Geometry: final body of the model. Coordinates: model frame, mm. Face numbers are marked on the shaded views. A direction names the side the tool comes from. Round coordinates to 2 decimals unless told otherwise and drop trailing zeros. Loops run counter-clockwise (first coordinate to the right, second up) from the corner with the lowest first, then second, coordinate; pieces in that order, holes last. Notation, with made-up numbers: M -10.5,-35.5 L -1.5,-35.5 A21 cw -1.5,-7.5 Z; hole C 30.5,-40 d4. An arc over 180 degrees is marked long. Answer as a JSON object with one key per item and string values.
```python
from build123d import *

# Parameters (mm, degrees)
F2_R = 1.6002
F3_R = 5.08


with BuildPart() as f1:
    # F0 (on Front) → F1 (revolve)
    with BuildSketch(Plane.XZ):
        Polygon((6.985, 12.7), (6.985, 0), (20.6375, 0), (20.6375, 17.4625), (19.05, 17.4625), (19.05, 19.05), (17.4625, 19.05), (17.4625, 12.7), align=None)
    revolve(axis=Axis((0, 0, 17.878274), (0, 0, 1)))

    # F2
    f2_edges = [f1.edges().sort_by_distance(p)[0] for p in [
        (-17.4625, 0, 12.7),
        (-20.6375, 0, 0),
    ]]
    fillet(f2_edges, radius=F2_R)

    # F3
    f3_edges = [f1.edges().sort_by_distance(p)[0] for p in [
        (-6.985, 0, 12.7),
    ]]
    fillet(f3_edges, radius=F3_R)


solid = f1.part
```
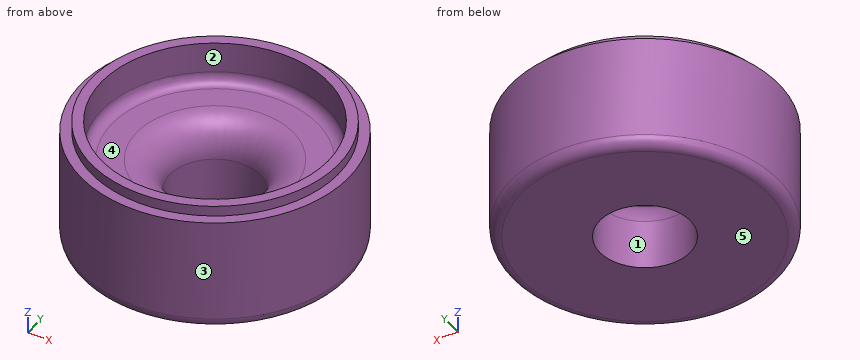
1) Cut plane D-D on z = 9. Return the cut outline in (x, y) (1 decimal), and give its area (3 significant figures).
Geometry results:
{"outline": "C 0,0 d41.3; hole C 0,0 d14.4", "area": "1,180 mm2"}
2) Set-up query: the marked faces 1 and 2. Return all of +Z, -Z, +X, -X, +Y, -Y with unobstructed straight access to the full face (end or side cutting, diameter ignored); none if empty.
Geometry results:
{"face 1": "+Z, -Z", "face 2": "+Z"}
3) Cut plane C-C on z = 5. Return the cut outline in (x, y) (1 decimal).
Geometry results:
{"outline": "C 0,0 d41.3; hole C 0,0 d14"}
4) First-contact query: pin 1 (1 mm diameter, centred on y = 13, z = 9.5, fed in from +X); pin 2 (1.5 mm diameter, centred on x = -10.5, z = 4.5, fed in from -Y); pin 3 (4 mm diameter, centred on x = 14, y = 5.5, fed in from +Z). Flat tips, straight axial feed; report the tip coordinate or a pass-through.
Geometry results:
{"pin 1": "x = 16.42", "pin 2": "y = -18.19", "pin 3": "z = 13.22"}
5) Line query: probe 1 along Y at (x, z) = (0, 16.75); probe 2 along Y at (x, z) = (0, 5.5) (1 decimal); probe 3 along Z at (x, y) = (-4.5, -12.5). Output: solid intervals per line, ascending.
Geometry results:
{"probe 1": "-20.64 to -17.46, 17.46 to 20.64", "probe 2": "-20.6 to -7, 7 to 20.6", "probe 3": "0 to 12.7"}
6) Pull-direction query (Y, two-part tool) for the marked faces 3, 4 and 5; classes: +Y half, -Y half, draft (parallel to the pull), parting line (faces both ways), or undercut.
Geometry results:
{"face 3": "parting line", "face 4": "undercut", "face 5": "draft"}
